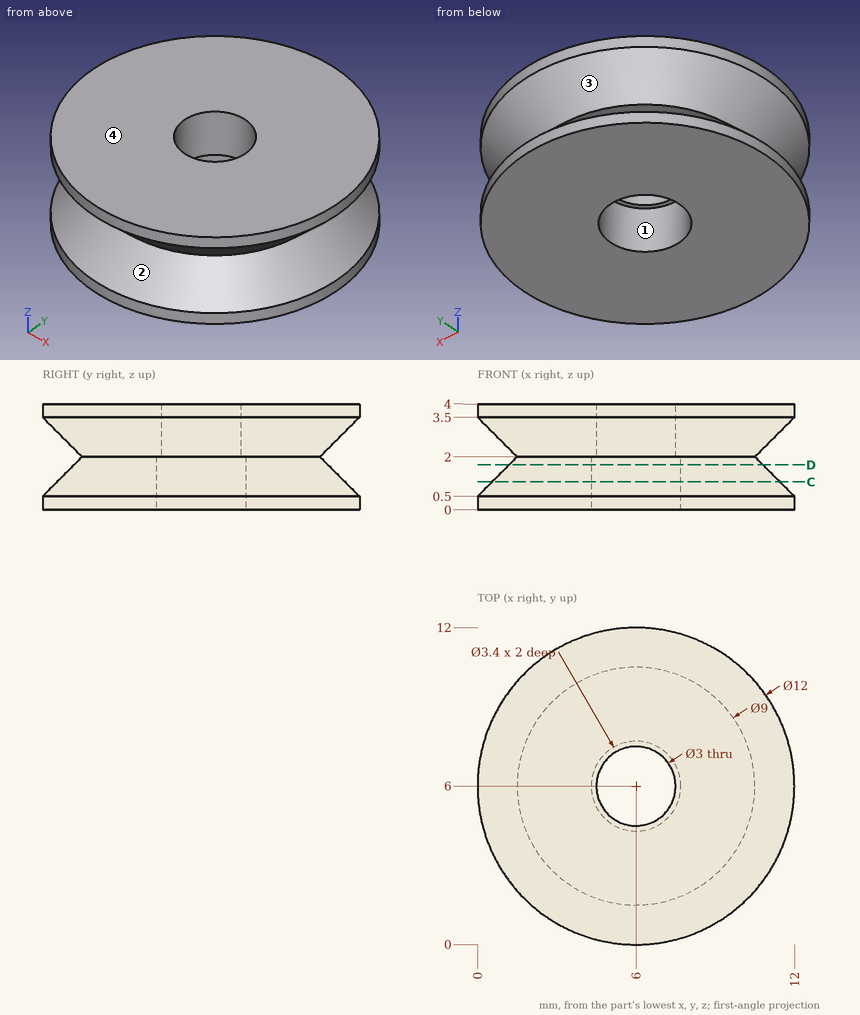
Job drawing, mm, ordinate dimensions from the low corner. One solid piece. Give positions to 0.01 mm unless a question says otherwise; leave off trailing zeros. Order: outer loops, then holes, each group sorted by start corner. A loop starts at its lowest first (then second) coordinate and runs counter-clockwise, first axis right, second up. Notation, with made-up numbers: (47.5, -25.75) - (100.5, -25.75) arc R20 cw to (100.5, -15.75) - close; hole circle Ø9 at (65, -6.5). An arc over 180 degrees is marked (long way). Answer in a Markdown table with one row per item.
1. Saw through at C-C, the plane z = 1.05. Give the cut face in (x, y).
Data:
| item | result |
|---|---|
| outline | circle Ø10.9 at (6, 6); hole circle Ø3.4 at (6, 6) |
2. Probe probe 1 along Z at (x, y) = (10.25, 4); probe 2 along Y at (x, z) = (6, 1.5); probe 3 along Y at (x, z) = (6, 1.15). List the from-to ranges inside material, lowest first. Write a range as [from, to].
Data:
| item | result |
|---|---|
| probe 1 | z = [0, 1.8], [2.2, 4] |
| probe 2 | y = [1, 4.3], [7.7, 11] |
| probe 3 | y = [0.65, 4.3], [7.7, 11.35] |
3. Flat gauge pins, fed straight in: pin 1 (2.5 mm diameter, centred on x = 6, y = 6, fed in from -Z); pin 2 (2 mm diameter, centred on x = 10.5, z = 2, fed in from +Y). Where does each tip first touch, or does it go through?
Data:
| item | result |
|---|---|
| pin 1 | passes through |
| pin 2 | stops at y = 9.59 |
4. Saw through at D-D, the plane z = 1.7. Give the cut face in (x, y), plus the area to 3 significant figures.
Data:
| item | result |
|---|---|
| outline | circle Ø9.6 at (6, 6); hole circle Ø3.4 at (6, 6) |
| area | 63.3 mm² |
5. Pull direction Z, two halves, no side cores. Call the marked faces 1, 2, 3 and 4: pulls with the +Z half, pulls with the -Z half, needs draft (parallel to the pull), parting line crosses it, or undercut.
Data:
| item | result |
|---|---|
| face 1 | needs draft |
| face 2 | undercut |
| face 3 | undercut |
| face 4 | pulls with the +Z half |
